Check sheet for the modelled part. Datum: model origin and axes. Units: mm. A direction names the side the tool comes from. Coordinates: 2 decimals unless noted, no trailing zeros. Write each loop counter-clockwise with the first axis right and the second up, starting at its lowest first coordinate (ties: lowest second). Pieces come first, ordered by that corner, then holes. Notation, with made-up numbers: (87.25, -19.5) - (107.25, -19.5) arc R12 cw to (107.25, -2.5) - close; hole circle Ø7 at (28, 8.25). An arc over 180 degrees is marked (long way). Use one line per item in the form item = value. Start each with the question number.
1. Draft check along Z on faces 1 (the face through (-0.86, 1.48, -6.6)), 2 (the face through (-25, 15, 0)), 3 (the face through (-23.521, 19.143, -1.301)). Enter one of: +Z half, -Z half, draft (parallel to the pull), parting line (faces both ways), or undercut.
2. Cross-section at A-A on x = -4.5. Record the boundary of the cut face in (y, z), then the cut area to 3 significant figures.
3. Cross-section at B-B on y = 25. Record the boundary of the cut face in (x, z), then the cut area to 3 significant figures.
4. Go/stop test with flat-tipped pins: pin 1 Ø4 at (x, z) = (-4.5, 0) entering from +Y; pin 2 Ø3 at (y, z) = (10, 4) entering from +X; pin 3 Ø6 at (x, y) = (-8, 7.5) entering from +Z; pin 4 Ø3 at (x, z) = (-18, -1) entering from -Y. Record where each tip stops, or that it passes through.
5. Tool access check on faces 4 (the face through (0, 2, 0)), 5 (the face through (-22, 16, 0)). Record the directions out of +Z, -Z, +X, -X, +Y, -Y that give a thin tool (end or side, any length) a straight path to the whole face; none if there is none.
6. Cross-section at C-C on z = 0. Record the boundary of the cut face in (x, y).
7. Scan lines: line 1 along Z through (x, y) = (-4.5, 1); line 2 along X through (y, z) = (32, 1.75); line 3 along Y through (x, z) = (-22.6, 0). Record each from-to range of solid material in increasing order.
8. Cross-section at D-D on z = -5.5. Record the boundary of the cut face in (x, y).
```python
from build123d import *

# Parameters (mm, degrees)
BASE_FLANGE1_DEPTH = 7.5
SKETCH6_R          = 6
CUT_EXTRUDE1_DEPTH = 43.86315434
SKETCH7_R          = 1.5
CUT_EXTRUDE2_DEPTH = 41.524683836
FILLET1_R          = 3


# Sheet-metal steps are written as plain solids
with BuildPart() as part:
    # Sketch1 → Base-Flange1 (new, symmetric)
    with BuildSketch(Plane.XY):
        with BuildLine():
            Line((0, 0), (-21.2634, 0))
            ThreePointArc((-21.2634, 0), (-23.905575199, 1.094424801), (-25, 3.7366))
            Line((-25, 3.7366), (-25, 34))
            Line((-25, 34), (-22, 34))
            Line((-22, 34), (-22, 3.7366))
            ThreePointArc((-22, 3.7366), (-21.784254855, 3.215745145), (-21.2634, 3))
            Line((-21.2634, 3), (0, 3))
            Line((0, 3), (0, 0))
        make_face()
    extrude(amount=BASE_FLANGE1_DEPTH, both=True)

    # Sketch6 → Cut-Extrude1 (cut, through all)
    with BuildSketch(Plane.ZY.offset(25)):
        with Locations((0, 25)):
            Circle(SKETCH6_R)
    extrude(amount=-CUT_EXTRUDE1_DEPTH, mode=Mode.SUBTRACT)

    # Sketch7 → Cut-Extrude2 (cut, through all)
    with BuildSketch(Plane(origin=(0, 3, 0), x_dir=(1, 0, 0), z_dir=(0, 1, 0))):
        with Locations(Location((-4.5, 0, 0), (0, 0, 180))):
            Circle(SKETCH7_R)
        with Locations(Location((-11.5, 0, 0), (0, 0, 180))):
            Circle(SKETCH7_R)
    extrude(amount=-CUT_EXTRUDE2_DEPTH, mode=Mode.SUBTRACT)

    # Fillet1
    fillet1_edges = [part.edges().sort_by_distance(p)[0] for p in [
        (0, 1.5, 7.5),
        (0, 1.5, -7.5),
        (-23.5, 34, 7.5),
        (-23.5, 34, -7.5),
    ]]
    fillet(fillet1_edges, radius=FILLET1_R)


solid = part.part
```
Final values:
q1.face_1 = -Z half
q1.face_2 = draft
q1.face_3 = undercut
q2.outline = (0, -7.5) - (3, -7.5) - (3, -1.5) - (0, -1.5) - close; (0, 1.5) - (3, 1.5) - (3, 7.5) - (0, 7.5) - close
q2.area = 36.0 mm²
q3.outline = (-25, -7.5) - (-22, -7.5) - (-22, -6) - (-25, -6) - close; (-25, 6) - (-22, 6) - (-22, 7.5) - (-25, 7.5) - close
q3.area = 9.00 mm²
q4.pin_1 = 3
q4.pin_2 = -22
q4.pin_3 = through
q4.pin_4 = 0
q5.face_4 = +Z, -Z, +X, +Y, -Y
q5.face_5 = +Z, -Z, +X, +Y
q6.outline = (-25, 3.74) arc R3.74 ccw to (-21.26, 0) - (-13, 0) - (-13, 3) - (-21.26, 3) arc R0.74 cw to (-22, 3.74) - (-22, 19) - (-25, 19) - close; (-25, 31) - (-22, 31) - (-22, 34) - (-25, 34) - close; (-10, 0) - (-6, 0) - (-6, 3) - (-10, 3) - close; (-3, 0) - (0, 0) - (0, 3) - (-3, 3) - close
q7.line_1 = -7.5 to -1.5, 1.5 to 7.5
q7.line_2 = -25 to -22
q7.line_3 = 0.25 to 19, 31 to 34
q8.outline = (-25, 3.74) arc R3.74 ccw to (-21.26, 0) - (-0.17, 0) - (-0.17, 3) - (-21.26, 3) arc R0.74 cw to (-22, 3.74) - (-22, 22.6) - (-25, 22.6) - close; (-25, 27.4) - (-22, 27.4) - (-22, 33.83) - (-25, 33.83) - close
